Geometry check sheet. Reference: drawing and pictorial views, mm from the part's lowest x, y, z. A direction names the side the tool comes from. Coordinates: 2 decimals unless noted, no trailing zeros. Loops run counter-clockwise (first coordinate to the right, second up) from the corner with the lowest first, then second, coordinate; pieces in that order, holes last. Notation, with made-up numbers: (-12.5, 48) - (39.5, 48) arc R35 ccw to (39.5, 86) - close; hole circle Ø7 at (-22.75, 54.5). An arc over 180 degrees is marked (long way). One line per item, written item: value.
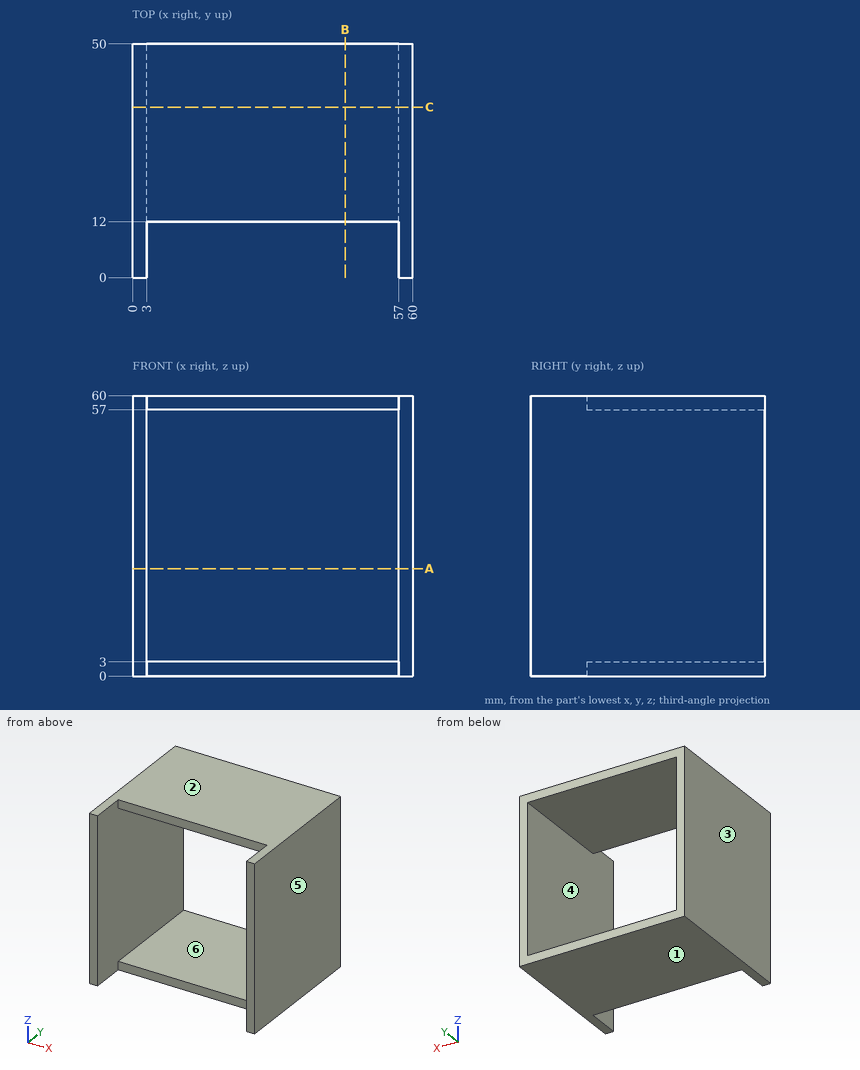
(1) Material ranges on probe 1 along X at (y, z) = (21, 44.5), recorded low to high. Write a range as from..to.
Reply:
probe 1: 0..3, 57..60
(2) Access from +Z, -Z, +X, -X, +Y, -Y to the whole of each face (thin tool, end or side, straight path). Record for the marked faces 5 and 6.
Reply:
face 5: +Z, -Z, +X, +Y, -Y
face 6: +Y, -Y
(3) Cross-section at C-C on y = 36.5. Record the cut outline in (x, z), and give its area (3 significant figures).
Reply:
outline: (0, 0) - (60, 0) - (60, 60) - (0, 60) - close; hole (3, 3) - (57, 3) - (57, 57) - (3, 57) - close
area: 684 mm2
(4) Cross-section at B-B on x = 45.5. Record the cut outline in (y, z), and give its area (3 significant figures).
Reply:
outline: (12, 0) - (50, 0) - (50, 3) - (12, 3) - close; (12, 57) - (50, 57) - (50, 60) - (12, 60) - close
area: 228 mm2
(5) Go/stop test with a flat-tipped pin: pin 1 Ø2.5 at (x, z) = (21.5, 59) entering from -Y. Record where the tip stops, or that it passes through.
Reply:
pin 1: y = 12
(6) Cross-section at A-A on z = 23. Record the cut outline in (x, y).
Reply:
outline: (0, 0) - (3, 0) - (3, 50) - (0, 50) - close; (57, 0) - (60, 0) - (60, 50) - (57, 50) - close
(7) Release check for a two-part mould opening along Z. For the marked faces 1, 2, 3 and 4 record: pulls with the +Z half, pulls with the -Z half, needs draft (parallel to the pull), parting line crosses it, or undercut.
Reply:
face 1: pulls with the -Z half
face 2: pulls with the +Z half
face 3: needs draft
face 4: undercut
